The listing builds one solid part. Answer for the finished solid, in the listing's coordinates (mm). A direction names the side the tool comes from. Coordinates: 2 decimals unless noted, no trailing zeros. Loops run counter-clockwise (first coordinate to the right, second up) from the corner with the lowest first, then second, coordinate; pieces in that order, holes last. Notation, with made-up numbers: (-4.5, -9.5) - (43.5, -9.5) arc R20 ccw to (43.5, -5.5) - close; hole circle Ø8 at (26.25, -26.75). An arc over 180 degrees is marked (long way). Put each result on its own line as item: value.
```python
from build123d import *

# Parameters (mm, degrees)
SKETCH1_W           = 16
SKETCH1_H           = 16
BOSS_EXTRUDE1_DEPTH = 16
SHELL1_T            = -1
SKETCH2_W           = 12
SKETCH2_H           = 12
CUT_EXTRUDE1_DEPTH  = 17
SKETCH3_W           = 12
SKETCH3_H           = 12
CUT_EXTRUDE3_DEPTH  = 7


with BuildPart() as part:
    # Sketch1 → Boss-Extrude1 (new body)
    with BuildSketch(Plane.XY):
        with Locations((8, 8)):
            Rectangle(SKETCH1_W, SKETCH1_H)
    extrude(amount=BOSS_EXTRUDE1_DEPTH)

    # Shell1
    shell1_openings = [part.faces().sort_by_distance(p)[0] for p in [
        (8, 0, 8),
    ]]
    offset(amount=SHELL1_T, openings=shell1_openings, kind=Kind.INTERSECTION)

    # Sketch2 → Cut-Extrude1 (cut, through all)
    with BuildSketch(Plane(origin=(0, 0, 0), x_dir=(-1, 0, 0), z_dir=(0, 0, -1))):
        with Locations((-8, 8)):
            Rectangle(SKETCH2_W, SKETCH2_H)
    extrude(amount=-CUT_EXTRUDE1_DEPTH, mode=Mode.SUBTRACT)

    # Sketch3 → Cut-Extrude3 (cut)
    with BuildSketch(Plane.ZY):
        with Locations((8, 8)):
            Rectangle(SKETCH3_W, SKETCH3_H)
    extrude(amount=-CUT_EXTRUDE3_DEPTH, mode=Mode.SUBTRACT)


solid = part.part
```
1) The part is cut by section A-A (x = 10.5). Give the vertices of the cut face in (y, z), and give its area (3 significant figures).
Found:
outline: (0, 0) - (2, 0) - (2, 1) - (0, 1) - close; (0, 15) - (2, 15) - (2, 16) - (0, 16) - close; (14, 0) - (16, 0) - (16, 16) - (14, 16) - (14, 15) - (15, 15) - (15, 1) - (14, 1) - close
area: 22.0 mm^2
2) For faces 4 (the face through (0.85, 0, 7.96)), 5 (the face through (15, 7, 8)), 6 (the face through (0.5, 14, 7.9)), 7 (the face through (0, 8, 15)), 8 (the face through (14, 7.9, 15.5)), determine the directions among +Z, -Z, +X, -X, +Y, -Y from which every point of the face is accessible in a straight line to the end or side of a thin tool.
Found:
face 4: +Z, -Z, +X, -X, -Y
face 5: -Y
face 6: -X
face 7: +Z, -Z, -X, +Y, -Y
face 8: +Z, -Z
3) This flat-tipped pin is pushed along its axis until it touches: pin 1 (2 mm diameter, centred on x = 12.5, z = 9, fed in from -Y). Where does it stop, or does it pass through?
Found:
pin 1: stops at y = 15
4) For a pull along Y with two mould halves and no side action, classify faces 1 (the face through (0.5, 7.9, 2)), 2 (the face through (1.7, 7.6, 15)), 3 (the face through (8, 15, 8)) as pulls with the +Y half, pulls with the -Y half, needs draft (parallel to the pull), parting line crosses it, or undercut.
Found:
face 1: undercut
face 2: needs draft
face 3: pulls with the -Y half
5) Straight lines are drawn through the part: L1, parallel to Z at x = 9.5, y = 0.5; L2, parallel to Y at x = 6.5, z = 6.75. For each, find the intervals that lie inside material, in ascending order. Write a range as [from, to].
Found:
L1: z = [0, 1], [15, 16]
L2: y = [15, 16]
6) The part is cut by section B-B (z = 13). Give the vertices of the cut face in (x, y).
Found:
outline: (0, 0) - (1, 0) - (1, 2) - (0, 2) - close; (0, 14) - (1, 14) - (1, 15) - (15, 15) - (15, 0) - (16, 0) - (16, 16) - (0, 16) - close
7) The part is cut by section C-C (y = 9). Give the vertices of the cut face in (x, z), and give its area (3 significant figures).
Found:
outline: (0, 0) - (2, 0) - (2, 1) - (1, 1) - (1, 2) - (0, 2) - close; (0, 14) - (1, 14) - (1, 15) - (2, 15) - (2, 16) - (0, 16) - close; (14, 0) - (16, 0) - (16, 16) - (14, 16) - (14, 15) - (15, 15) - (15, 1) - (14, 1) - close
area: 24.0 mm^2
